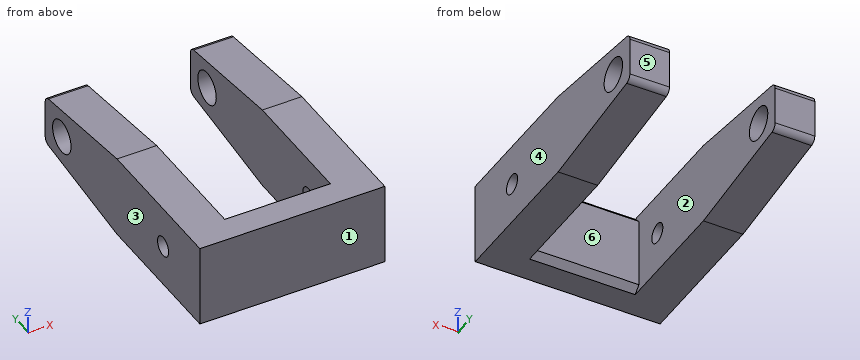
from build123d import *

# Parameters (mm, degrees)
SKETCH1_R           = 3
SKETCH1_R_2         = 5
BOSS_EXTRUDE1_DEPTH = 12
SKETCH3_W           = 25
SKETCH3_H           = 10
BOSS_EXTRUDE2_DEPTH = 16
CHAMFER1_SIZE       = 2


with BuildPart() as part:
    # Sketch1 → Boss-Extrude1 (new body)
    with BuildSketch(Plane(origin=(0, 0, 0), x_dir=(0, 0, -1), z_dir=(1, 0, 0))):
        with BuildLine():
            Line((-12.5, 45), (-7.723804022, 82.254328632))
            ThreePointArc((-7.723804022, 82.254328632), (-7.061279266, 83.501442184), (-5.740040692, 84))
            Line((-5.740040692, 84), (5.740040692, 84))
            ThreePointArc((5.740040692, 84), (7.061279266, 83.501442184), (7.723804022, 82.254328632))
            Line((7.723804022, 82.254328632), (12.5, 45))
            Line((12.5, 45), (12.5, 0))
            Line((12.5, 0), (-12.5, 0))
            Line((-12.5, 0), (-12.5, 45))
        make_face()
        with Locations((0, 20)):
            Circle(SKETCH1_R, mode=Mode.SUBTRACT)
        with Locations((0, 75)):
            Circle(SKETCH1_R_2, mode=Mode.SUBTRACT)
    extrude(amount=BOSS_EXTRUDE1_DEPTH)

    # Sketch3 → Boss-Extrude2 (add)
    with BuildSketch(Plane.ZY):
        with Locations((0, 5)):
            Rectangle(SKETCH3_W, SKETCH3_H)
    extrude(amount=BOSS_EXTRUDE2_DEPTH)

    # Mirror2: part across plane


with BuildPart() as part_1:
    add(part.part)
    add(part.part.mirror(Plane(origin=(-16, 0, 0), x_dir=(0, 0, 1), z_dir=(1, 0, 0))))

    # Chamfer1
    chamfer1_edges = [part_1.edges().sort_by_distance(p)[0] for p in [
        (-16, 10, -12.5),
        (-16, 10, 12.5),
    ]]
    chamfer(chamfer1_edges, length=CHAMFER1_SIZE)


solid = part_1.part
The listing builds one solid part. Answer for the finished solid, in the listing's coordinates (mm). Face numbers are marked on the shaded views. A direction names the side the tool comes from. Coordinates: 2 decimals unless noted, no trailing zeros. Write each loop counter-clockwise with the first axis right and the second up, starting at its lowest first coordinate (ties: lowest second). Pieces come first, ordered by that corner, then holes. Notation, with made-up numbers: M -12,-19.5 L 11,-19.5 A17 ccw 11,2.5 Z; hole C 5.5,-36.5 d8. An arc over 180 degrees is marked long. Put each result on its own line as item: value. Start each with the question number.
1. A flat-ended cylindrical pin translates along its axis: P1, Ø8, axis at x = -6.5, z = 2.5, coming from the +Y side. Find the tip coordinate at first contact, or state that the pin passes through.
2. A cutting plane is placed at B-B on z = 0. Write down the section's boundary in (x, y), then the cut area to 3 significant figures.
3. A cutting plane is placed at C-C on x = -38. Write down the section's boundary in (y, z).
4. A cutting plane is placed at D-D on z = 9.25. Write down the section's boundary in (x, y).
5. For a pull along X with two mould halves and no side action, classify the marked faces 1, 2, 3 and 4 as pulls with the +X half, pulls with the -X half, needs draft (parallel to the pull), parting line crosses it, or undercut.
6. Consider line 1 (Y direction, x = -40.5, z = 0); line 2 (X direction, y = 44, z = 10); line 3 (Y direction, x = -7.5, z = 2.75). Determine where each line is inside the solid, lowest interval first. Write a range as from..to.
7. Which of the six approach directions +Z, -Z, +X, -X, +Y, -Y give full straight-line access (tool end or side, diameter ignored) to the marked faces 5 and 6?
8. A cutting plane is placed at A-A on y = 20. Write down the section's boundary in (x, z), then the cut area to 3 significant figures.
Resolved:
1. P1: stops at y = 10
2. outline: M -44,0 L 12,0 L 12,17 L 0,17 L 0,10 L -32,10 L -32,17 L -44,17 Z; M -44,23 L -32,23 L -32,70 L -44,70 Z; M -44,80 L -32,80 L -32,84 L -44,84 Z; M 0,23 L 12,23 L 12,70 L 0,70 Z; M 0,80 L 12,80 L 12,84 L 0,84 Z
2. area: 1,950 mm2
3. outline: M 0,-12.5 L 45,-12.5 L 82.25,-7.72 A2 ccw 84,-5.74 L 84,5.74 A2 ccw 82.25,7.72 L 45,12.5 L 0,12.5 Z; hole C 20,0 d6; hole C 75,0 d10
4. outline: M -44,0 L 12,0 L 12,70.35 L 0,70.35 L 0,10 L -32,10 L -32,70.35 L -44,70.35 Z
5. face 1: needs draft
5. face 2: undercut
5. face 3: pulls with the -X half
5. face 4: pulls with the +X half
6. line 1: y = 0..17, 23..70, 80..84
6. line 2: x = -44..-32, 0..12
6. line 3: y = 0..10
7. face 5: +Z, -Z, +X, -X, +Y
7. face 6: +Z, -Z, +Y
8. outline: M -44,-12.5 L -32,-12.5 L -32,-3 L -44,-3 Z; M -44,3 L -32,3 L -32,12.5 L -44,12.5 Z; M 0,-12.5 L 12,-12.5 L 12,-3 L 0,-3 Z; M 0,3 L 12,3 L 12,12.5 L 0,12.5 Z
8. area: 456 mm2
